The model under review builds one solid part; all positions refer to its coordinate system, in mm. Face numbers are marked on the shaded views. A direction names the side the tool comes from. Coordinates: 2 decimals unless noted, no trailing zeros. Loops run counter-clockwise (first coordinate to the right, second up) from the corner with the lowest first, then second, coordinate; pieces in that order, holes last. Notation, with made-up numbers: M -39,44.5 L 7,44.5 A16 cw 7,59.5 Z; hole C 3,-20.5 d1. An arc over 180 degrees is marked long. Use CSV: the item, a comma, the result in double quotes. Start each with the question number.
1. Tool access review of the marked faces 4, 5, 6, 7 and 8: name each direction out of +Z, -Z, +X, -X, +Y, -Y from which nothing blocks a thin tool from reaching the whole face with its end or side.
2. Add section B-B, the plane y = 33. State how many separate pieces and enclosed holes the cut face has, then the cut area to 3 significant figures.
3. Clearance check with flat-ended pins moving along their axes: P1, Ø6, axis at x = 13, y = 39.5, coming from the -Z side; P2, Ø1, axis at y = 32, z = -61.5, coming from the +X side; P3, Ø10, axis at y = 44, z = -28.5, coming from the +X side. State where each tip first meets the part, or that it passes through.
4. For L1, parallel to Z at x = -1.5, y = 40.5; L2, parallel to Z at x = -7, y = 19.5; L3, parallel to Z at x = -29, y = 14.5, list the stretches that pass through material, from the lowest coordinate up.
5. Draft analysis for pull direction X (two halves, no side actions). For the marked faces 1, 2 and 3, state which applies: +X half, -X half, draft (parallel to the pull), parting line (faces both ways), or undercut.
6. Add section A-A, the plane z = -65. Write out the cut boundary in (x, y).
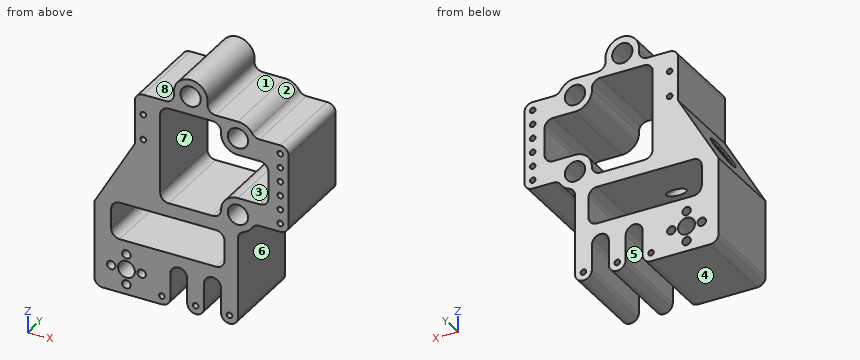
from build123d import *

# Parameters (mm, degrees)
F2_DEPTH  = 50
F0_R      = 6
F0_R_2    = 5
F3_DEPTH  = 50.001
F4_D      = 3.3
F5_D      = 5
F7_R      = 10
F8_DEPTH  = 1
F9_D      = 10.8
F9_DEPTH  = 18.75
F9_START  = 1
F9_TIP    = 3.2446473427
F10_D     = 6
F10_DEPTH = 18.75
F10_START = 21.1920655
F10_TIP   = 1.8025818571


with BuildPart() as f2:
    # F1 (on Front) → F2 (new body)
    with BuildSketch(Plane.XZ):
        with BuildLine():
            ThreePointArc((-2, -75), (3, -80), (8, -75))
            ThreePointArc((8, -75), (3, -70), (-2, -75))
        make_face()
        with BuildLine():
            ThreePointArc((-2, -75), (3, -70), (8, -75))
            Line((8, -75), (8, -60))
            ThreePointArc((8, -60), (13, -55), (18, -60))
            Line((18, -60), (18, -75))
            ThreePointArc((18, -75), (23, -80), (28, -75))
            Line((28, -75), (28, -27.1421356237))
            ThreePointArc((28, -27.1421356237), (28.9175170954, -24.2553842778), (31.3333333333, -22.4280904158))
            ThreePointArc((31.3333333333, -22.4280904158), (34.2415418806, -20.8130119002), (36.4590516936, -18.3333333333))
            ThreePointArc((36.4590516936, -18.3333333333), (38.2733480828, -16.6220248211), (40.6885775404, -16))
            Line((40.6885775404, -16), (53, -16))
            ThreePointArc((53, -16), (56.5355339059, -14.5355339059), (58, -11))
            Line((58, -11), (58, 31))
            ThreePointArc((58, 31), (56.5355339059, 34.5355339059), (53, 36))
            Line((53, 36), (40.6885775404, 36))
            ThreePointArc((40.6885775404, 36), (38.2733480828, 36.6220248211), (36.4590516936, 38.3333333333))
            ThreePointArc((36.4590516936, 38.3333333333), (32.8304589154, 41.7559503577), (28, 43))
            Line((28, 43), (14.8660687473, 43))
            ThreePointArc((14.8660687473, 43), (11.1022054838, 44.708597057), (9.9107124982, 48.6666666667))
            ThreePointArc((9.9107124982, 48.6666666667), (0, 60), (-9.9107124982, 48.6666666667))
            ThreePointArc((-9.9107124982, 48.6666666667), (-11.1022054838, 44.708597057), (-14.8660687473, 43))
            Line((-14.8660687473, 43), (-28, 43))
            ThreePointArc((-28, 43), (-31.5355339059, 41.5355339059), (-33, 38))
            Line((-33, 38), (-33, 12))
            Line((-33, 12), (-57, -29.5692193817))
            Line((-57, -29.5692193817), (-57, -75))
            ThreePointArc((-57, -75), (-55.5355339059, -78.5355339059), (-52, -80))
            Line((-52, -80), (-17, -80))
            ThreePointArc((-17, -80), (-13.4644660941, -78.5355339059), (-12, -75))
            Line((-12, -75), (-12, -60))
            ThreePointArc((-12, -60), (-7, -55), (-2, -60))
            Line((-2, -60), (-2, -75))
        make_face()
        with BuildLine():
            ThreePointArc((-47, -31), (-45.5355339059, -27.4644660941), (-42, -26))
            Line((-42, -26), (15, -26))
            ThreePointArc((15, -26), (18.5355339059, -27.4644660941), (20, -31))
            Line((20, -31), (20, -43))
            ThreePointArc((20, -43), (18.5355339059, -46.5355339059), (15, -48))
            Line((15, -48), (-42, -48))
            ThreePointArc((-42, -48), (-45.5355339059, -46.5355339059), (-47, -43))
            Line((-47, -43), (-47, -31))
        make_face(mode=Mode.SUBTRACT)
        with BuildLine():
            Line((-18, -13), (-18, 34))
            ThreePointArc((-18, 34), (-16.5355339059, 37.5355339059), (-13, 39))
            Line((-13, 39), (13, 39))
            ThreePointArc((13, 39), (16.5355339059, 37.5355339059), (18, 34))
            Line((18, 34), (18, 33))
            ThreePointArc((18, 33), (20.9289321881, 25.9289321881), (28, 23))
            Line((28, 23), (41, 23))
            ThreePointArc((41, 23), (44.5355339059, 21.5355339059), (46, 18))
            Line((46, 18), (46, 2))
            ThreePointArc((46, 2), (44.5355339059, -1.5355339059), (41, -3))
            Line((41, -3), (28, -3))
            ThreePointArc((28, -3), (20.9289321881, -5.9289321881), (18, -13))
            ThreePointArc((18, -13), (16.5355339059, -16.5355339059), (13, -18))
            Line((13, -18), (-13, -18))
            ThreePointArc((-13, -18), (-16.5355339059, -16.5355339059), (-18, -13))
        make_face(mode=Mode.SUBTRACT)
    extrude(amount=-F2_DEPTH)

    # F0 (on Front) → F3 (cut, through all)
    with BuildSketch(Plane.XZ):
        with Locations((0, 50)):
            Circle(F0_R)
        with Locations((28, 33)):
            Circle(F0_R)
        with Locations((28, -13)):
            Circle(F0_R)
        with Locations((-38, -65)):
            Circle(F0_R_2)
    extrude(amount=-F3_DEPTH, mode=Mode.SUBTRACT)

    # F4 (through all)
    with Locations(Plane.XZ):
        with Locations((53, 31), (53, 22.6), (53, 14.2), (53, 5.8), (53, -2.6), (53, -11), (-28, 16), (-28, 31), (-17, -75), (3, -75), (23, -75)):
            Hole(F4_D / 2)

    # F5 (through all)
    with Locations(Plane.XZ):
        with Locations((-47, -65), (-38, -56), (-29, -65), (-38, -74)):
            Hole(F5_D / 2)

    # F7 (on face) → F8 (cut)
    with BuildSketch(Plane(origin=(-29.9461524227, 0, 17.2894191624), x_dir=(0, -1, 0), z_dir=(-0.8660254038, 0, 0.5))):
        with Locations((-25, -31.5166604984)):
            Circle(F7_R)
    extrude(amount=-F8_DEPTH, mode=Mode.SUBTRACT)

    # F9
    # its depths count from where the whole tool has entered the part; down to there all is cleared
    with Locations(Plane(origin=(-29.9461524227, 0, 17.2894191624), x_dir=(0, -1, 0), z_dir=(-0.8660254038, 0, 0.5)).offset(-F9_START)):
        with Locations((-25, -31.5166604984)):
            Hole(F9_D / 2, depth=F9_DEPTH)
            with Locations((0, 0, -(F9_DEPTH + F9_TIP / 2))):  # 118° drill point
                Cone(0, F9_D / 2, F9_TIP, mode=Mode.SUBTRACT)

    # F10
    # its depths count from where the whole tool has entered the part; down to there all is cleared
    with Locations(Plane(origin=(-29.9461524227, 0, 17.2894191624), x_dir=(0, -1, 0), z_dir=(-0.8660254038, 0, 0.5))):
        with Locations((-25, -31.5166604984)):
            Hole(F10_D / 2, depth=F10_START)
    with Locations(Plane(origin=(-29.9461524227, 0, 17.2894191624), x_dir=(0, -1, 0), z_dir=(-0.8660254038, 0, 0.5)).offset(-F10_START)):
        with Locations((-25, -31.5166604984)):
            Hole(F10_D / 2, depth=F10_DEPTH)
            with Locations((0, 0, -(F10_DEPTH + F10_TIP / 2))):  # 118° drill point
                Cone(0, F10_D / 2, F10_TIP, mode=Mode.SUBTRACT)


solid = f2.part
Computed:
1,face 4,"-Z, +X, -X, +Y, -Y"
1,face 5,"-Z, +Y, -Y"
1,face 6,"-Z, +X, +Y, -Y"
1,face 7,"+Y, -Y"
1,face 8,"+Z, -X, +Y, -Y"
2,separate pieces,"1"
2,enclosed holes,"21"
2,area,"5,810 mm^2"
3,P1,"stops at z = -56"
3,P2,"stops at x = 28"
3,P3,"stops at x = 29.57"
4,L1,"z = -77.18 to -48, -26 to -18, 39 to 44.19, 55.81 to 59.89"
4,L2,"z = -55 to -48, -26 to -18, 39 to 57.14"
4,L3,"z = -80 to -67.5, -62.5 to -48, -26 to 14.69, 17.31 to 29.69, 32.31 to 42.9"
5,face 1,"draft"
5,face 2,"+X half"
5,face 3,"undercut"
6,outline,"M -57,0 L -49.5,0 L -49.5,50 L -57,50 Z; M -44.5,0 L -43,0 L -43,50 L -44.5,50 Z; M -33,0 L -31.5,0 L -31.5,50 L -33,50 Z; M -26.5,0 L -12,0 L -12,50 L -26.5,50 Z; M -2,0 L 8,0 L 8,50 L -2,50 Z; M 18,0 L 28,0 L 28,50 L 18,50 Z"
